For this review, use the dimensioned drawing (mm, ordinates from the lowest corner) and the shaded views. A direction names the side the tool comes from. Give positions to 0.01 mm unless a question says otherwise; leave off trailing zeros. Order: outer loops, then holes, each group sorted by start corner. A loop starts at its lowest first (then second) coordinate and runs counter-clockwise, first axis right, second up. Notation, with made-up numbers: M -4,-5 L 34,-5 A16 cw 34,25 Z; hole C 5,1.5 d1. An arc over 180 degrees is marked long. One line per question, with ' | ' between items. Start each with the question number.
1. We need section C-C on x = 5.5. Write out the cut boundary in (y, z), then the cut area to 4 significant figures.
2. For the marked faces 4 and 5, list the 3-axis set-ups (+Z, -Z, +X, -X, +Y, -Y) from which the entire face can be reached by the end or side of a thin tool; tool diameter is ignored.
3. We need section D-D on z = 17. Write out the cut boundary in (x, y), then the cut area to 3 significant figures.
4. We need section A-A on z = 5. Write out the cut boundary in (x, y), then the cut area to 3 significant figures.
5. Wall thickness on L1, parallel to Z at x = 15.5, y = 10.5; L2, parallel to X at y = 24, z = 2; L3, parallel to X at y = 48, z = 5: over which ranges is each line inside the solid? List them lowest first.
6. We need section B-B on y = 27.5. Write out the cut boundary in (x, z), then the cut area to 3 significant figures.
7. The part is to be moulded in two halves that separate along X. For the marked faces 1, 2 and 3, say which applies: +X half, -X half, draft (parallel to the pull), parting line (faces both ways), or undercut.
8. Insertion check: P1, Ø6, axis at y = 9, z = 7.5, coming from the -X side; P2, Ø4, axis at x = 21, y = 28.5, coming from the -Z side; P3, Ø2, axis at y = 6, z = 25.5, coming from the +X side. Each pin has a flat end and moves straight along its axis. Give the tip position at first contact, or say it passes through.
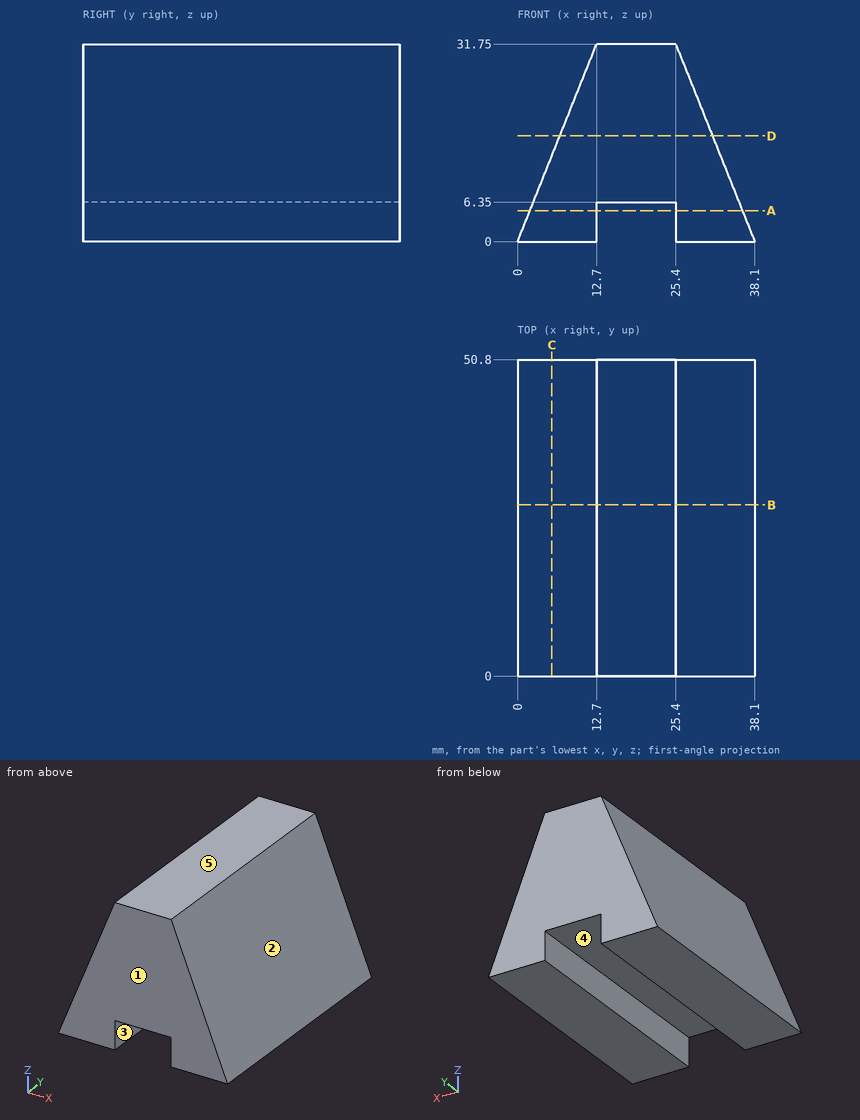
Entries:
1) outline: M 0,0 L 50.8,0 L 50.8,13.75 L 0,13.75 Z | area: 698.5 mm^2
2) face 4: -Z, +Y, -Y | face 5: +Z, +X, -X, +Y, -Y
3) outline: M 6.8,0 L 31.3,0 L 31.3,50.8 L 6.8,50.8 Z | area: 1,240 mm^2
4) outline: M 2,0 L 12.7,0 L 12.7,50.8 L 2,50.8 Z; M 25.4,0 L 36.1,0 L 36.1,50.8 L 25.4,50.8 Z | area: 1,090 mm^2
5) L1: z = 6.35 to 31.75 | L2: x = 0.8 to 12.7, 25.4 to 37.3 | L3: x = 2 to 12.7, 25.4 to 36.1
6) outline: M 0,0 L 12.7,0 L 12.7,6.35 L 25.4,6.35 L 25.4,0 L 38.1,0 L 25.4,31.75 L 12.7,31.75 Z | area: 726 mm^2
7) face 1: draft | face 2: +X half | face 3: undercut
8) P1: stops at x = 1.8 | P2: stops at z = 6.35 | P3: stops at x = 28.3
